The drawing under review shows one solid part. Ordinate dimensions are in mm from its lowest x, y, z. A direction names the side the tool comes from. Give positions to 0.01 mm unless a question says otherwise; leave off trailing zeros. Loops run counter-clockwise (first coordinate to the right, second up) from the corner with the lowest first, then second, coordinate; pieces in that order, holes last. Notation, with made-up numbers: M 85.25,2.25 L 113.25,2.25 A22 ccw 113.25,30.25 Z; hole C 17.5,5.5 d10. An arc over 180 degrees is marked long. One line per item, written item: value. Start each with the question number.
Q1. For the marked faces 1 and 2, list the 3-axis set-ups (+Z, -Z, +X, -X, +Y, -Y) from which the entire face can be reached by the end or side of a thin tool; tool diameter is ignored.
Q2. We need section C-C on x = 9.25. Write out the cut boundary in (y, z).
Q3. For pin 1 (4 mm diameter, centred on y = 11, z = 2, fed in from -X); pin 2 (2.5 mm diameter, centred on x = 2.5, y = 4.5, fed in from +Z); pin 3 (2.5 mm diameter, centred on x = 2.64, y = 4.1, fed in from +Z); pin 4 (1.5 mm diameter, centred on x = 7.5, z = 6, fed in from +Y), all flat-tipped, find the tip position at first contact; note any pin that passes through.
Q4. We need section D-D on y = 3. Write out the cut boundary in (x, z).
Q5. We need section B-B on x = 6.1. Write out the cut boundary in (y, z), plus the area to 3 significant figures.
Q6. We need section A-A on y = 6.1. Write out the cut boundary in (x, z).
Q7. To check wall thickness, follow line 1 along Y through (x, z) = (6.1, 6.25); line 2 along Y through (x, z) = (6.5, 1.5); line 3 along X through (y, z) = (6, 1.75). State the ranges of each line that lie inside material, in increasing order. Write a range as from..to.
Q8. Mouldability with a two-part tool opening along X and no side actions: class the marked faces 3, 4 and 5 as released by +X, released by -X, zero draft, split by the parting line, or undercut.
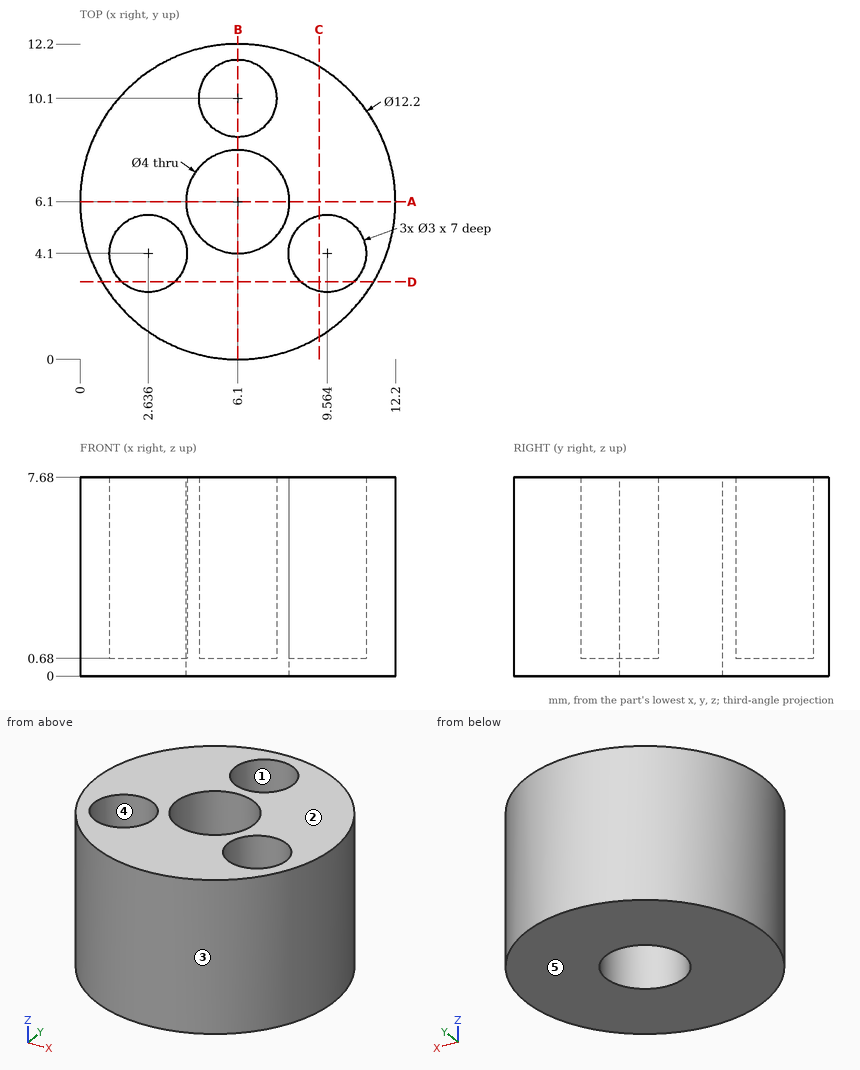
Solved:
1. face 1: +Z
1. face 2: +Z, +X, -X, +Y, -Y
2. outline: M 0.88,0 L 11.32,0 L 11.32,7.68 L 5.57,7.68 L 5.57,0.68 L 2.63,0.68 L 2.63,7.68 L 0.88,7.68 Z
3. pin 1: x = 0.73
3. pin 2: z = 7.68
3. pin 3: z = 0.68
3. pin 4: y = 12.17
4. outline: M 0.85,0 L 11.35,0 L 11.35,7.68 L 10.58,7.68 L 10.58,0.68 L 8.54,0.68 L 8.54,7.68 L 3.66,7.68 L 3.66,0.68 L 1.62,0.68 L 1.62,7.68 L 0.85,7.68 Z
5. outline: M 0,0 L 4.1,0 L 4.1,7.68 L 0,7.68 Z; M 8.1,0 L 12.2,0 L 12.2,7.68 L 11.6,7.68 L 11.6,0.68 L 8.6,0.68 L 8.6,7.68 L 8.1,7.68 Z
5. area: 42.0 mm2
6. outline: M 0,0 L 4.1,0 L 4.1,7.68 L 0,7.68 Z; M 8.1,0 L 12.2,0 L 12.2,7.68 L 8.1,7.68 Z
7. line 1: 0..4.1, 8.1..8.6, 11.6..12.2
7. line 2: 0.01..4.14, 8.06..8.65, 11.55..12.19
7. line 3: 0..4.1, 8.1..12.2
8. face 3: split by the parting line
8. face 4: undercut
8. face 5: zero draft
